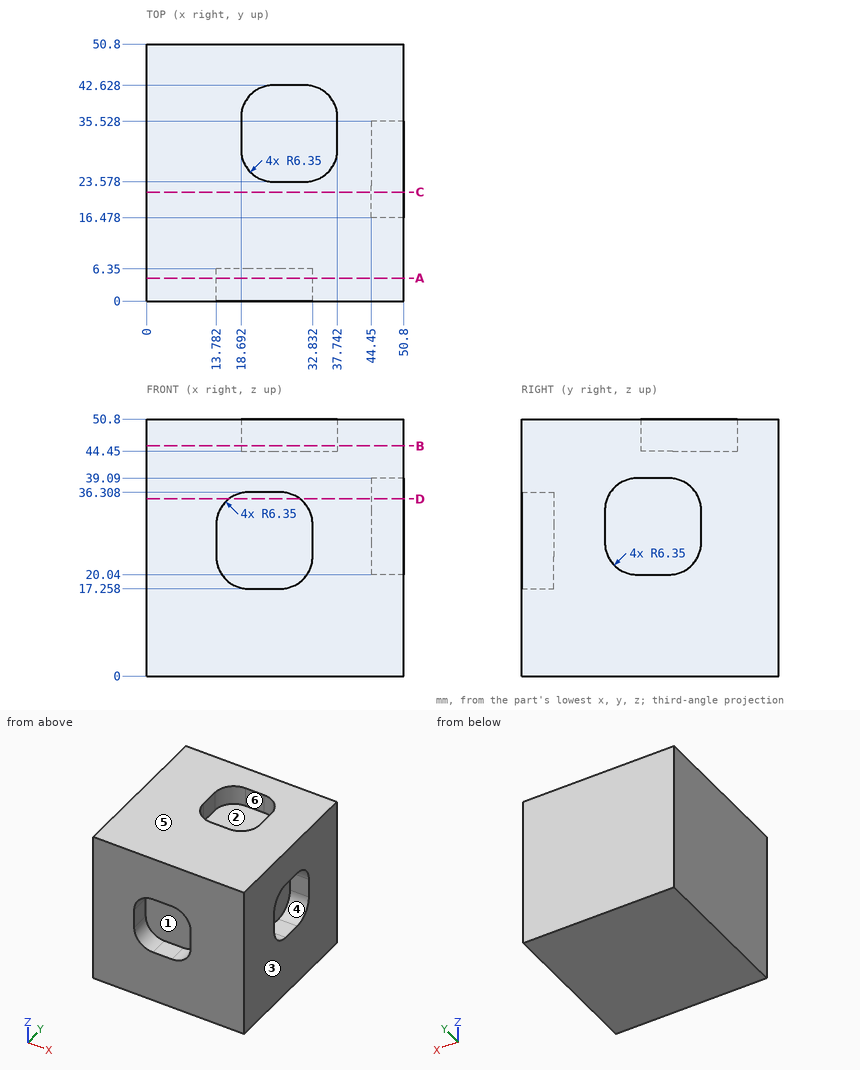
Check sheet for the drawn part. Datum: minimum x, y, z corner. Units: mm. A direction names the side the tool comes from. Coordinates: 2 decimals unless noted, no trailing zeros. Order: outer loops, then holes, each group sorted by start corner. A loop starts at its lowest first (then second) coordinate and runs counter-clockwise, first axis right, second up. Notation, with made-up numbers: M 69.5,68 L 108.5,68 A34 cw 108.5,100 Z; hole C 82.5,-37.75 d4. An arc over 180 degrees is marked long. One line per question, with ' | ' between items. Start each with the question number.
Item 1: Cross-section at D-D on z = 35. Enter the section's corners in (x, y), then the cut area to 3 significant figures.
Item 2: Gauge pin test, flat end, axial feed: pin 1 (15 mm diameter, centred on x = 30, y = 32.5, fed in from +Z). Record the tip position at first contact, or that the pin passes through.
Item 3: Cross-section at A-A on y = 4.5. Enter the section's corners in (x, z), then the cut area to 3 significant figures.
Item 4: Material ranges on L1, parallel to X at y = 33, z = 46.5; L2, parallel to X at y = 29.5, z = 24; L3, parallel to Y at x = 17.5, z = 20.5, recorded low to high. Write a range as [from, to].
Item 5: Cross-section at C-C on y = 21.5. Enter the section's corners in (x, z).
Item 6: Set-up check for the marked faces 4, 5 and 6: record each of +Z, -Z, +X, -X, +Y, -Y from which the full face is reachable in a straight line by a thin tool's end or side.
Item 7: Draft check along Z on the marked faces 1, 2 and 3. Enter one of: pulls with the +Z half, pulls with the -Z half, needs draft (parallel to the pull), parting line crosses it, or undercut.
Item 8: Cross-section at B-B on z = 45.5. Enter the section's corners in (x, y), then the cut area to 3 significant figures.
Findings:
1) outline: M 0,0 L 16.27,0 L 16.27,6.35 L 30.34,6.35 L 30.34,0 L 50.8,0 L 50.8,16.89 L 44.45,16.89 L 44.45,35.11 L 50.8,35.11 L 50.8,50.8 L 0,50.8 Z | area: 2,380 mm²
2) pin 1: stops at z = 44.45
3) outline: M 0,0 L 50.8,0 L 50.8,50.8 L 0,50.8 Z; hole M 13.78,23.61 A6.35 ccw 20.13,17.26 L 26.48,17.26 A6.35 ccw 32.83,23.61 L 32.83,29.96 A6.35 ccw 26.48,36.31 L 20.13,36.31 A6.35 ccw 13.78,29.96 Z | area: 2,250 mm²
4) L1: x = [0, 18.69], [37.74, 50.8] | L2: x = [0, 44.45] | L3: y = [6.35, 50.8]
5) outline: M 0,0 L 50.8,0 L 50.8,20.18 L 44.45,20.18 L 44.45,38.95 L 50.8,38.95 L 50.8,50.8 L 0,50.8 Z
6) face 4: +X | face 5: +Z, +X, -X, +Y, -Y | face 6: +Z
7) face 1: undercut | face 2: pulls with the +Z half | face 3: needs draft
8) outline: M 0,0 L 50.8,0 L 50.8,50.8 L 0,50.8 Z; hole M 18.69,29.93 A6.35 ccw 25.04,23.58 L 31.39,23.58 A6.35 ccw 37.74,29.93 L 37.74,36.28 A6.35 ccw 31.39,42.63 L 25.04,42.63 A6.35 ccw 18.69,36.28 Z | area: 2,250 mm²
